```python
from build123d import *

# Parameters (mm, degrees)
ESBO_O1_R                  = 20
ESBO_O1_R_2                = 0.75
RESSALTO_EXTRUS_O1_DEPTH   = 25
ESBO_O2_W                  = 4
ESBO_O2_H                  = 42.07133093
ESBO_O2_W_2                = 15.138637908
ESBO_O2_H_2                = 40
ESBO_O2_W_3                = 12.263470243
CORTE_EXTRUS_O1_DEPTH      = 20
ESBO_O3_R                  = 2
CORTE_EXTRUS_O2_DEPTH      = 20
CORTE_EXTRUS_O2_DEPTH_BACK = 20
FILETE1_R                  = 4


with BuildPart() as part:
    # Esboço1 → Ressalto-extrusão1 (new body)
    with BuildSketch(Plane(origin=(0, 0, 0), x_dir=(1, 0, 0), z_dir=(0, 1, 0))):
        Circle(ESBO_O1_R)
        Circle(ESBO_O1_R_2, mode=Mode.SUBTRACT)
    extrude(amount=RESSALTO_EXTRUS_O1_DEPTH)

    # Esboço2 → Corte-extrusão1 (cut)
    with BuildSketch(Plane(origin=(0, 0, 0), x_dir=(1, 0, 0), z_dir=(0, 1, 0))):
        with Locations((0, -0.26404601)):
            Rectangle(ESBO_O2_W, ESBO_O2_H)
        with Locations((-17.569318954, 0)):
            Rectangle(ESBO_O2_W_2, ESBO_O2_H_2)
        with Locations((16.131735122, -0.26404601)):
            Rectangle(ESBO_O2_W_3, ESBO_O2_H)
    extrude(amount=CORTE_EXTRUS_O1_DEPTH, mode=Mode.SUBTRACT)

    # Esboço3 → Corte-extrusão2 (cut, two sides)
    with BuildSketch(Plane(origin=(0, 0, 0), x_dir=(0, 0, -1), z_dir=(1, 0, 0))) as corte_extrus_o2_sk:
        with Locations((-8.660254038, 10)):
            Circle(ESBO_O3_R)
        with Locations((8.660254038, 10)):
            Circle(ESBO_O3_R)
    extrude(amount=CORTE_EXTRUS_O2_DEPTH, mode=Mode.SUBTRACT)
    extrude(corte_extrus_o2_sk.sketch, amount=-CORTE_EXTRUS_O2_DEPTH_BACK, mode=Mode.SUBTRACT)

    # Filete1
    filete1_edges = [part.edges().sort_by_distance(p)[0] for p in [
        (-10, 20, 0),
        (10, 20, 0),
    ]]
    fillet(filete1_edges, radius=FILETE1_R)


solid = part.part
```
Here's how the part is built. I have some questions about the finished solid (model axes, mm). A direction names the side the tool comes from. Coordinates: 2 decimals unless noted, no trailing zeros. Write each loop counter-clockwise with the first axis right and the second up, starting at its lowest first coordinate (ties: lowest second). Pieces come first, ordered by that corner, then holes. Notation, with made-up numbers: (81, -2) - (122, -2) arc R36 cw to (122, 36) - close; hole circle Ø1 at (34, 33.25). An arc over 180 degrees is marked (long way). One line per item, written item: value.
1) On a 3-axis mill with a long thin cutter (end or side, diameter ignored), from which of +Z, -Z, +X, -X, +Y, -Y can I reach the whole of each face in a straight line? I mean faces 1 (the flat face through (2, 10, 0)), 2 (the flat face through (16, 20, 0)), 3 (the flat face through (-10, 8, 0)). Say none if no direction works.
Model answer:
face 1: +Z, -Z, -Y
face 2: +Z, -Z, +X, -Y
face 3: +Z, -Z, -X, -Y
2) Suppose I cut it at A-A on y = 10. Write out the boundary of the cut face in (x, z), and give its area (3 significant figures).
Model answer:
outline: (-10, -17.32) arc R20 ccw to (-2, -19.9) - (-2, -10.66) - (-10, -10.66) - close; (-10, -6.66) - (-2, -6.66) - (-2, 6.66) - (-10, 6.66) - close; (-10, 10.66) - (-2, 10.66) - (-2, 19.9) arc R20 ccw to (-10, 17.32) - close; (2, -19.9) arc R20 ccw to (10, -17.32) - (10, -10.66) - (2, -10.66) - close; (2, -6.66) - (10, -6.66) - (10, 6.66) - (2, 6.66) - close; (2, 10.66) - (10, 10.66) - (10, 17.32) arc R20 ccw to (2, 19.9) - close
area: 478 mm²
3) I need wall thicknesses on line 1 along X through (y, z) = (11, 2.5); line 2 along Z through (x, y) = (0, 22.95); line 3 along Z through (x, y) = (7.25, 10). Which ranges of each line are inside material? Lowest first, please.
Model answer:
line 1: x = -10 to -2, 2 to 10
line 2: z = -20 to -0.75, 0.75 to 20
line 3: z = -18.64 to -10.66, -6.66 to 6.66, 10.66 to 18.64
4) We'd pull the mould along X, two halves only. Please class faces 4 (the cylindrical face through (-0.75, 22.46, -0.03)), 5 (the flat face through (6, 0, 0)), 6 (the flat face through (10, 8, 0)): pulls with the +X half, pulls with the -X half, needs draft (parallel to the pull), parting line crosses it, or undercut.
Model answer:
face 4: undercut
face 5: needs draft
face 6: pulls with the +X half
5) Suppose I cut it at D-D on x = 0. Write out the boundary of the cut face in (y, z), and give its area (4 significant figures).
Model answer:
outline: (20, -20) - (25, -20) - (25, -0.75) - (20, -0.75) - close; (20, 0.75) - (25, 0.75) - (25, 20) - (20, 20) - close
area: 192.5 mm²
6) Suppose I cut it at B-B on z = 0. Write out the boundary of the cut face in (x, y).
Model answer:
outline: (-20, 20) - (-14, 20) arc R4 cw to (-10, 16) - (-10, 0) - (-2, 0) - (-2, 20) - (-0.75, 20) - (-0.75, 25) - (-20, 25) - close; (0.75, 20) - (2, 20) - (2, 0) - (10, 0) - (10, 16) arc R4 cw to (14, 20) - (20, 20) - (20, 25) - (0.75, 25) - close
7) I'm going to push flat-ended pins straight in: P1, Ø4, axis at x = -11, y = 14, coming from the -Z side; P2, Ø6, axis at x = -7, z = -1, coming from the -Y side; P3, Ø5, axis at y = 8.5, z = -0.5, coming from the +X side; P4, Ø6.5, axis at x = 17, z = -6, coming from the -Y side. Where does each tip first touch, or does it pass through?
Model answer:
P1: stops at z = -17.86
P2: stops at y = 0
P3: stops at x = 10
P4: stops at y = 19.99
8) Suppose I cut it at C-C on y = 2.25. Write out the boundary of the cut face in (x, z).
Model answer:
outline: (-10, -17.32) arc R20 ccw to (-2, -19.9) - (-2, 19.9) arc R20 ccw to (-10, 17.32) - close; (2, -19.9) arc R20 ccw to (10, -17.32) - (10, 17.32) arc R20 ccw to (2, 19.9) - close
